The figure shows three views and two pictorial views of one solid part (mm, origin at its lowest corner). Answer the questions. A direction names the side the tool comes from. Coordinates: 2 decimals unless noted, no trailing zeros. Write each loop counter-clockwise with the first axis right and the second up, starting at its lowest first coordinate (ties: lowest second). Pieces come first, ordered by that corner, then holes. Notation, with made-up numbers: M 81,45.5 L 85,45.5 A24 cw 85,69.5 Z; hole C 33.5,89 d2. An arc over 180 degrees is marked long. Write item = value, one per line.
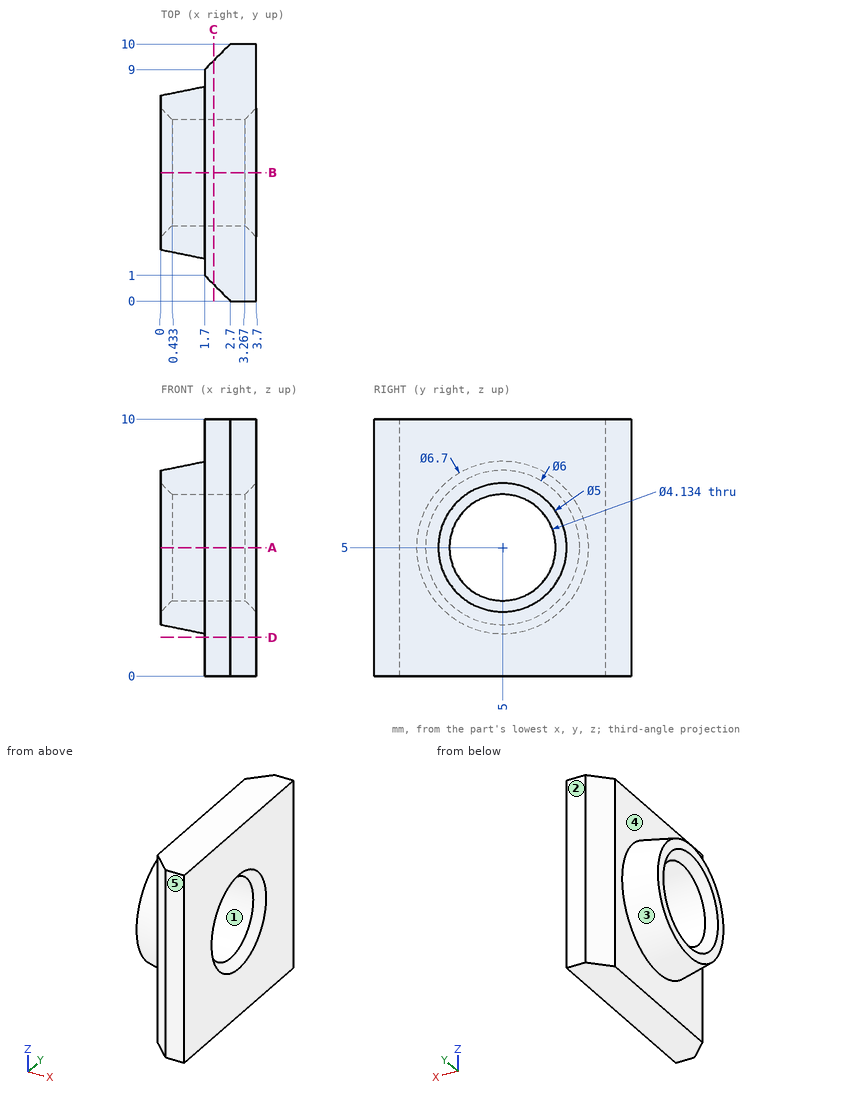
Item 1: Consider line 1 along Z through (x, y) = (1.95, 5); line 2 along X through (y, z) = (1.75, 1.5); line 3 along Y through (x, z) = (0.4, 6.25). Determine where each line is inside the solid, lowest interval first. Write a range as from..to.
Worked answers:
line_1 = 0..2.93, 7.07..10
line_2 = 1.7..3.7
line_3 = 2.18..3.31, 6.69..7.82
Item 2: Find section A-A (z = 5). Determine the outline of the cut face in (x, y), and give its area (3 significant figures).
Worked answers:
outline = M 0,2 L 1.7,1.65 L 1.7,1 L 2.7,0 L 3.7,0 L 3.7,2.5 L 3.27,2.93 L 0.43,2.93 L 0,2.5 Z; M 0,7.5 L 0.43,7.07 L 3.27,7.07 L 3.7,7.5 L 3.7,10 L 2.7,10 L 1.7,9 L 1.7,8.35 L 0,8 Z
area = 14.1 mm²
Item 3: Find section D-D (z = 1.5). Determine the outline of the cut face in (x, y).
Worked answers:
outline = M 1.7,1 L 2.7,0 L 3.7,0 L 3.7,10 L 2.7,10 L 1.7,9 Z
Item 4: Find section C-C (x = 2.05). Determine the outline of the cut face in (y, z), and give its area (3 significant figures).
Worked answers:
outline = M 0.65,0 L 9.35,0 L 9.35,10 L 0.65,10 Z; hole C 5,5 d4.13
area = 73.6 mm²
Item 5: Find section B-B (y = 5). Determine the outline of the cut face in (x, z).
Worked answers:
outline = M 0,2 L 1.7,1.65 L 1.7,0 L 3.7,0 L 3.7,2.5 L 3.27,2.93 L 0.43,2.93 L 0,2.5 Z; M 0,7.5 L 0.43,7.07 L 3.27,7.07 L 3.7,7.5 L 3.7,10 L 1.7,10 L 1.7,8.35 L 0,8 Z
Item 6: Which of the six approach directions +Z, -Z, +X, -X, +Y, -Y give full straight-line access (tool end or side, diameter ignored) to the marked faces 4 and 5?
Worked answers:
face_4 = -X
face_5 = +Z, -Z, +X, -X, -Y
Item 7: For a pull along Y with two mould halves and no side action, classify the marked faces 1, 2 and 3 as released by +Y, released by -Y, zero draft, split by the parting line, or undercut.
Worked answers:
face_1 = undercut
face_2 = released by +Y
face_3 = split by the parting line
